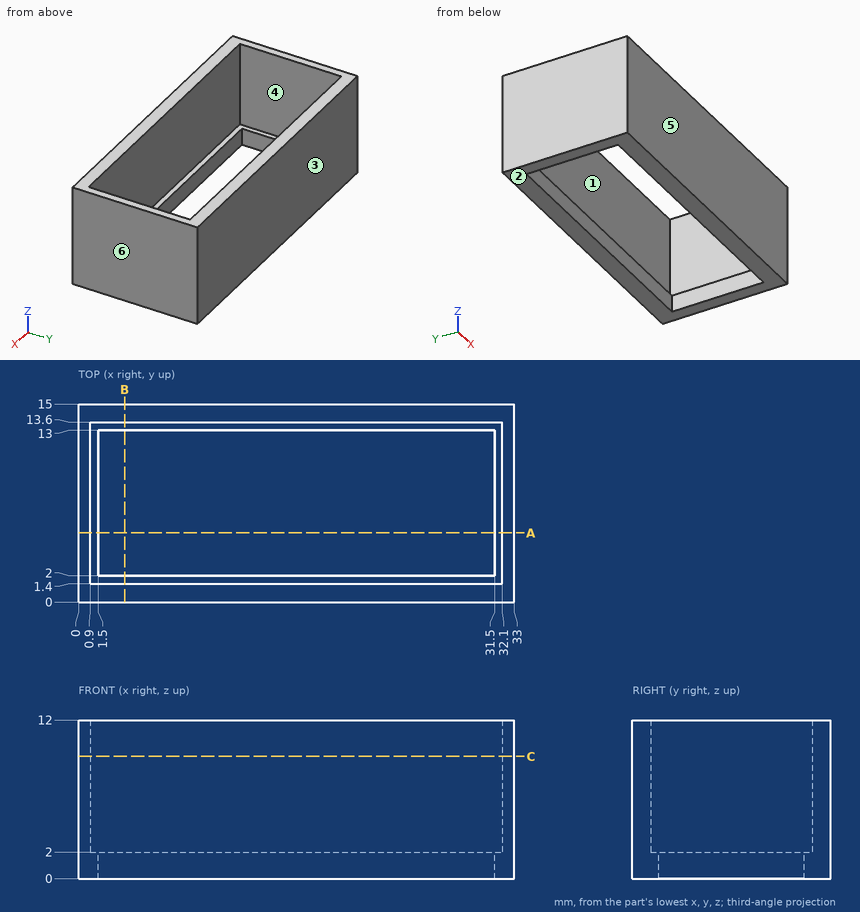
Input: dimensioned drawing with shaded views. Units: mm. Origin: part minimum x, y, z. A direction names the side the tool comes from. Give positions to 0.01 mm unless a question says otherwise; leave off trailing zeros. Write each loop counter-clockwise with the first axis right and the second up, starting at its lowest first coordinate (ties: lowest second). Pieces come first, ordered by that corner, then holes.
1. Draft query along Y for the marked faces 3, 4, 5 and 6. Return one class per face: released by +Y, released by -Y, zero draft, split by the parting line, or undercut.
2. Section query A-A, the plane y = 5.25. Return loops of the section in (x, z).
3. Section query C-C, the plane z = 9.25. Return loops of the section in (x, y), then the cut area to 3 significant figures.
4. Reachability of the marked faces 1 and 2 from +Z, -Z, +X, -X, +Y, -Y: full face, straight path, thin tool, end or side. Return the list, or none.
5. Line query: probe 1 along Y at (x, z) = (16, 2.25); probe 2 along X at (y, z) = (13.25, 8.5); probe 3 along Y at (x, z) = (4, 1.5). Output: solid intervals per line, ascending.
6. Section query B-B, the plane x = 3.5. Return loops of the section in (y, z).
Computed:
1. face 3: released by +Y
1. face 4: undercut
1. face 5: released by -Y
1. face 6: zero draft
2. outline: (0, 0) - (1.5, 0) - (1.5, 2) - (0.9, 2) - (0.9, 12) - (0, 12) - close; (31.5, 0) - (33, 0) - (33, 12) - (32.1, 12) - (32.1, 2) - (31.5, 2) - close
3. outline: (0, 0) - (33, 0) - (33, 15) - (0, 15) - close; hole (0.9, 1.4) - (32.1, 1.4) - (32.1, 13.6) - (0.9, 13.6) - close
3. area: 114 mm2
4. face 1: +Z
4. face 2: -Z, +X, -X, +Y, -Y
5. probe 1: y = 0 to 1.4, 13.6 to 15
5. probe 2: x = 0 to 0.9, 32.1 to 33
5. probe 3: y = 0 to 2, 13 to 15
6. outline: (0, 0) - (2, 0) - (2, 2) - (1.4, 2) - (1.4, 12) - (0, 12) - close; (13, 0) - (15, 0) - (15, 12) - (13.6, 12) - (13.6, 2) - (13, 2) - close
